For this review, take the finished solid that the model builds, in its own axes (mm). A direction names the side the tool comes from. Coordinates: 2 decimals unless noted, no trailing zeros. Write each loop counter-clockwise with the first axis right and the second up, starting at its lowest first coordinate (ties: lowest second). Pieces come first, ordered by that corner, then holes. Notation, with made-up numbers: (85, 89) - (101, 89) arc R14 ccw to (101, 111) - close; hole circle Ø2 at (21.25, 81). An arc over 180 degrees is marked (long way). Use one line per item in the form item = value. Start each with the question number.
1) Tool access review of faces 1 (the cylindrical face through (-2.2, 2, 4.6)), 2 (the cylindrical face through (-1.73, -7.81, 0.49)): name each direction out of +Z, -Z, +X, -X, +Y, -Y from which nothing blocks a thin tool from reaching the whole face with its end or side.
2) We need section D-D (z = 2.5). Give the boundary of the cut face in (x, y) (3 decimals), plus the area to 3 significant figures.
3) For L1, parallel to Z at x = 0.75, y = -5; L2, parallel to Y at x = -2.5, z = 7.5, list the stretches that pass through material, from the lowest coordinate up. Write a range as from..to.
4) We need section A-A (y = 0). Give the boundary of the cut face in (x, z) (3 decimals).
5) Insertion check: P1, Ø4, axis at x = -0.5, y = 6, coming from the +Z side; P2, Ø4, axis at y = 4, z = 4.5, coming from the -X side; P3, Ø4, axis at y = 5.5, z = 5, coming from the -X side. Each pin has a flat end and moves straight along its axis. Give the tip position at first contact, or say it passes through.
6) We need section C-C (z = 0.75). Give the boundary of the cut face in (x, y).
```python
from build123d import *

# Parameters (mm, degrees)
F0_R     = 8
F1_DEPTH = 1
F3_R     = 8
F4_DEPTH = 1
F5_R     = 2.975
F6_DEPTH = 7.4


with BuildPart() as f1:
    # F0 (on Top) → F1 (new body)
    with BuildSketch(Plane.XY):
        with Locations((-0.1634992032, 0.8891506742)):
            Circle(F0_R)
    extrude(amount=F1_DEPTH)


with BuildPart() as f4:
    # F3 (on Top) → F4 (new body)
    with BuildSketch(Plane.XY):
        Circle(F3_R)
    extrude(amount=F4_DEPTH)

    # F5 (on face) → F6 (join)
    with BuildSketch(Plane.XY.offset(1)):
        Circle(F5_R)
    extrude(amount=F6_DEPTH)


solid = f4.part
```
Determined:
q1.face_1 = +Z
q1.face_2 = +Z, -Z
q2.outline = circle Ø5.95 at (0, 0)
q2.area = 27.8 mm²
q3.L1 = 0..1
q3.L2 = -1.61..1.61
q4.outline = (-8, 0) - (8, 0) - (8, 1) - (2.975, 1) - (2.975, 8.4) - (-2.975, 8.4) - (-2.975, 1) - (-8, 1) - close
q5.P1 = 1
q5.P2 = -2.2
q5.P3 = through
q6.outline = circle Ø16 at (0, 0)
